Check sheet for the modelled part. Datum: model origin and axes. Units: mm. A direction names the side the tool comes from. Round coordinates to 2 decimals unless told otherwise and drop trailing zeros. Write each loop counter-clockwise with the first axis right and the second up, starting at its lowest first coordinate (ties: lowest second). Pieces come first, ordered by that corner, then holes.
Item 1: Section check A-A, the plane z = -2.8. Record the cut outline in (x, y), plus the area to 3 significant figures.
Item 2: Depth check by flat-ended pin: pin 1 (1.5 mm diameter, centred on y = 5, z = -2.5, fed in from -X); pin 2 (2 mm diameter, centred on x = -17.5, y = 4, fed in from -Z). Enter the tip coordinate at first touch or a pass-through.
Item 3: Section check C-C, the plane y = 3.25. Record the cut outline in (x, z), plus the area to 3 significant figures.
Item 4: Set-up check for faces 5 (the flat face through (-27, 6.1, -3)), 6 (the flat face through (-2, 9, -2)): record each of +Z, -Z, +X, -X, +Y, -Y from which the full face is reachable in a straight line by a thin tool's end or side.
Item 5: Section check B-B, the plane x = -15. Record the cut outline in (y, z), plus the area to 3 significant figures.
Item 6: Section check D-D, the plane y = 12.25. Record the cut outline in (x, z).
Item 7: Release check for a two-part mould opening along Y. For faces 1 (the flat face through (-27, 9, 0)), 2 (the flat face through (-27, 18.05, -2)), 3 (the flat face through (-27, 0, -2)), 4 (the flat face through (-27, 4, -1.95)) record: pulls with the +Y half, pulls with the -Y half, needs draft (parallel to the pull), parting line crosses it, or undercut.
Item 8: Material ranges on line 1 along Y through (x, z) = (-14, -3.25); line 2 along Z through (x, y) = (-39, 5); line 3 along X through (y, z) = (9, -3.2), recorded low to high.
Autodesk Inventor part; units mm, degrees
ref_plane "XZ Plane" through (0, 0, 0) normal (0, 1, 0) x (-1, 0, 0)
ref_plane "XY Plane" through (0, 0, 0) normal (0, 0, 1) x (1, 0, 0)
sketch "Sketch1" plane through (0, 0, 0) normal (0, 1, 0) x (-1, 0, 0)
  line L0 (0, 0) -> (54, 0)
  line L1 (4, -4) -> (50, -4)
  line L2 (0, -4) -> (50, -4) construction
  line L3 (50, -4) -> (54, 0)
  line L4 (0, 0) -> (4, -4)
  dimension "d0" = 54
  dimension "d1" = 4
  dimension "d3" = 0
extrude "Extrusion1" add sketch "Sketch1" along normal blind 17
sketch "Sketch2" plane through (-4, 0, -4) normal (0, 0, -1) x (-1, 0, 0)
  line L0 (-4, 0) -> (-4, 17)
  line L1 (50, 0) -> (50, 17)
  line L2 (-4, 2) -> (50, 2)
  line L3 (50, 2) -> (50, 6.1)
  line L4 (50, 6.1) -> (-4, 6.1)
  line L5 (-4, 6.1) -> (-4, 2)
  line L6 (0, 0) -> (46, 0)
  point P0 (-4, 6.1)
  dimension "d6" = 4.1
  dimension "d7" = 2
sketch "Sketch3" plane through (0, 17, 0) normal (0, 1, 0) x (1, 0, 0)
  line L0 (-50, 4) -> (-54, 0)
  line L1 (-54, 0) -> (0, 0)
  line L2 (0, 0) -> (-4, 4)
  line L3 (-4, 4) -> (-50, 4)
extrude "Extrusion2" add sketch "Sketch3" along normal blind 1.05
extrude "Extrusion3" cut sketch "Sketch2" against normal blind 2.05
ref_plane "Work Plane1" through (-27, 0, 0) normal (1, 0, 0) x (0, 1, 0)
properties part number "PDMS Chamber-Mold-V8-Left_Right-Wall Steven"
Values found:
1. outline: (-51.2, 0) - (-2.8, 0) - (-2.8, 2) - (-51.2, 2) - close; (-51.2, 6.1) - (-2.8, 6.1) - (-2.8, 18.05) - (-51.2, 18.05) - close
1. area: 675 mm2
2. pin 1: stops at x = -52.25
2. pin 2: stops at z = -1.95
3. outline: (-54, 0) - (-52.05, -1.95) - (-1.95, -1.95) - (0, 0) - close
3. area: 101 mm2
4. face 5: -Z, +X, -X
4. face 6: -Z, +X, +Y, -Y
5. outline: (0, -4) - (2, -4) - (2, -1.95) - (6.1, -1.95) - (6.1, -4) - (18.05, -4) - (18.05, 0) - (0, 0) - close
5. area: 63.8 mm2
6. outline: (-54, 0) - (-50, -4) - (-4, -4) - (0, 0) - close
7. face 1: needs draft
7. face 2: pulls with the +Y half
7. face 3: pulls with the -Y half
7. face 4: undercut
8. line 1: y = 0 to 2, 6.1 to 18.05
8. line 2: z = -1.95 to 0
8. line 3: x = -50.8 to -3.2
